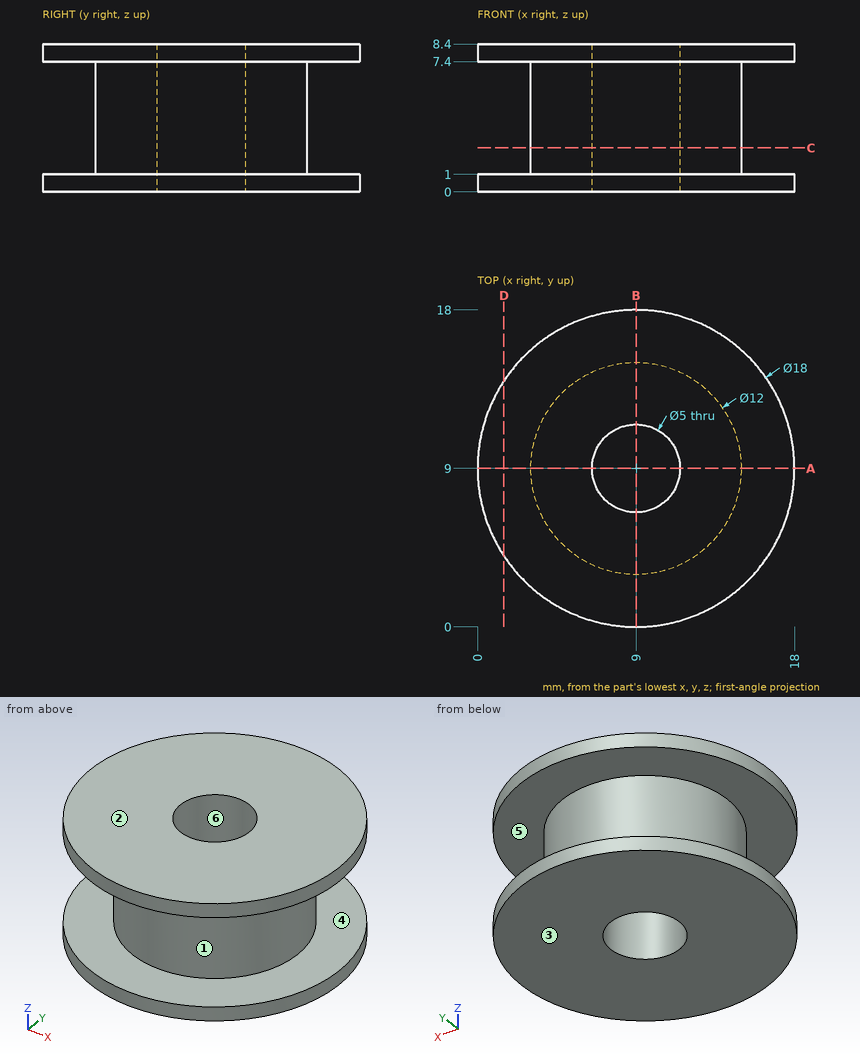
Could you check a few things on this drawing? It's one solid part, dimensions in mm from its lowest x, y, z. A direction names the side the tool comes from. Round coordinates to 2 decimals unless told otherwise and drop trailing zeros. Loops run counter-clockwise (first coordinate to the right, second up) from the corner with the lowest first, then second, coordinate; pieces in that order, holes last.
Q1. Thinking about a two-plate mould opening in Z: for the marked faces 3, 4, 5 and 6, which applies, pulls with the +Z half, pulls with the -Z half, needs draft (parallel to the pull), parting line crosses it, or undercut?
Q2. On a 3-axis mill with a long thin cutter (end or side, diameter ignored), from which of +Z, -Z, +X, -X, +Y, -Y can I reach the whole of each face in a straight line? I mean the marked faces 1 and 2. Say none if no direction works.
Q3. Please list where these lines run through material, in increasing order: L1, parallel to Y at x = 9, z = 4.25; L2, parallel to Z at x = 3, y = 11.5; L3, parallel to Y at x = 11.25, z = 6.75.
Q4. I want a section at D-D (x = 1.5). Write out the boundary of the cut face in (y, z).
Q5. I want a section at A-A (y = 9). Write out the boundary of the cut face in (x, z).
Q6. For P1, Ø1.5, axis at y = 5.5, z = 3.5, coming from the +X side; P2, Ø1.5, axis at y = 10, z = 2.5, coming from the +X side; P3, Ø3, axis at x = 15, z = 4.5, coming from the -Y side, each with a flat end and sliding along its axis, tell me the tip position at first contact or that it passes through.
Q7. I want a section at C-C (z = 2.5). Write out the boundary of the cut face in (x, y), and give its area (3 significant figures).
Answer below:
1. face 3: pulls with the -Z half
1. face 4: undercut
1. face 5: undercut
1. face 6: needs draft
2. face 1: none
2. face 2: +Z, +X, -X, +Y, -Y
3. L1: y = 3 to 6.5, 11.5 to 15
3. L2: z = 0 to 1, 7.4 to 8.4
3. L3: y = 3.44 to 7.91, 10.09 to 14.56
4. outline: (4.03, 0) - (13.97, 0) - (13.97, 1) - (4.03, 1) - close; (4.03, 7.4) - (13.97, 7.4) - (13.97, 8.4) - (4.03, 8.4) - close
5. outline: (0, 0) - (6.5, 0) - (6.5, 8.4) - (0, 8.4) - (0, 7.4) - (3, 7.4) - (3, 1) - (0, 1) - close; (11.5, 0) - (18, 0) - (18, 1) - (15, 1) - (15, 7.4) - (18, 7.4) - (18, 8.4) - (11.5, 8.4) - close
6. P1: stops at x = 14.33
6. P2: stops at x = 14.99
6. P3: stops at y = 5.03
7. outline: circle Ø12 at (9, 9); hole circle Ø5 at (9, 9)
7. area: 93.5 mm2
